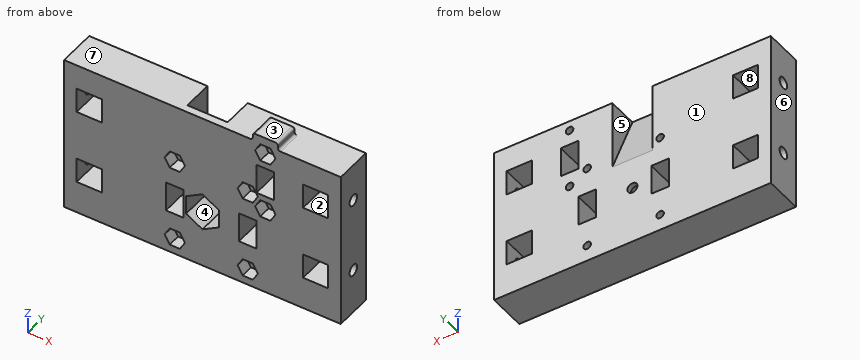
from build123d import *

# Parameters (mm, degrees)
CROQUIS1_W              = 80
CROQUIS1_H              = 60
CROQUIS1_R              = 1.5
CROQUIS1_W_2            = 7
CROQUIS1_H_2            = 25
CROQUIS1_W_3            = 10
CROQUIS1_H_3            = 20
CROQUIS1_H_4            = 10
CROQUIS1_W_4            = 5
CROQUIS1_H_5            = 6.5
SALIENTE_EXTRUIR1_DEPTH = 15
CORTAR_EXTRUIR1_DEPTH   = 5
CROQUIS3_R              = 1.5
CORTAR_EXTRUIR2_DEPTH   = 25
CROQUIS6_R              = 1.5
CORTAR_EXTRUIR3_DEPTH   = 25
CROQUIS8_W              = 15
CROQUIS8_H              = 17.838651154
CROQUIS8_R              = 2
SALIENTE_EXTRUIR2_DEPTH = 2
CORTAR_EXTRUIR4_START   = -55
CORTAR_EXTRUIR4_DEPTH   = 8
CROQUIS10_R             = 1.5
CROQUIS10_W             = 7
CROQUIS10_H             = 12
CORTAR_EXTRUIR5_DEPTH   = 16
CROQUIS12_W             = 110
CROQUIS12_H             = 15
SALIENTE_EXTRUIR3_DEPTH = 3
CORTAR_EXTRUIR6_DEPTH   = 5
SALIENTE_EXTRUIR4_DEPTH = 10
CROQUIS15_R             = 2.25
CORTAR_EXTRUIR7_DEPTH   = 10
CROQUIS16_R             = 2.25
CORTAR_EXTRUIR8_DEPTH   = 10


with BuildPart() as part:
    # Croquis1 → Saliente-Extruir1 (new body)
    with BuildSketch(Plane(origin=(0, 0, 0), x_dir=(1, 0, 0), z_dir=(0, 1, 0))):
        with Locations((0, -10)):
            Rectangle(CROQUIS1_W, CROQUIS1_H)
        with Locations(Location((18, -16.5, 0), (0, 0, 270))):
            Circle(CROQUIS1_R, mode=Mode.SUBTRACT)
        with Locations(Location((-11, -16.5, 0), (0, 0, 270))):
            Circle(CROQUIS1_R, mode=Mode.SUBTRACT)
        with Locations(Location((18, 16.5, 0), (0, 0, 270))):
            Circle(CROQUIS1_R, mode=Mode.SUBTRACT)
        with Locations(Location((-11, 16.5, 0), (0, 0, 270))):
            Circle(CROQUIS1_R, mode=Mode.SUBTRACT)
        with Locations((18, 0)):
            Rectangle(CROQUIS1_W_2, CROQUIS1_H_2, mode=Mode.SUBTRACT)
        Polygon((6.495190528, 3.75), (0, 7.5), (-6.495190528, 3.75), (-6.495190528, -3.75), (0, -7.5), (6.495190528, -3.75), align=None, mode=Mode.SUBTRACT)
        with Locations((-11, 0)):
            Rectangle(CROQUIS1_W_2, CROQUIS1_H_2, mode=Mode.SUBTRACT)
        with Locations((-45, -10)):
            Rectangle(CROQUIS1_W_3, CROQUIS1_H_3)
        with Locations((-45, -35)):
            Rectangle(CROQUIS1_W_3, CROQUIS1_H_4)
        with Locations((-52.5, -10)):
            Rectangle(CROQUIS1_W_4, CROQUIS1_H)
        with Locations((-45, 15)):
            Rectangle(CROQUIS1_W_3, CROQUIS1_H_4)
        with Locations((45, 15)):
            Rectangle(CROQUIS1_W_3, CROQUIS1_H_4)
        with Locations((52.5, -10)):
            Rectangle(CROQUIS1_W_4, CROQUIS1_H)
        with Locations((45, -10)):
            Rectangle(CROQUIS1_W_3, CROQUIS1_H_3)
        with Locations((45, -35)):
            Rectangle(CROQUIS1_W_3, CROQUIS1_H_4)
        with Locations((-11, 9.25)):
            Rectangle(CROQUIS1_W_2, CROQUIS1_H_5)
        with Locations((-11, -9.25)):
            Rectangle(CROQUIS1_W_2, CROQUIS1_H_5)
        with Locations((18, 9.25)):
            Rectangle(CROQUIS1_W_2, CROQUIS1_H_5)
        with Locations((18, -9.25)):
            Rectangle(CROQUIS1_W_2, CROQUIS1_H_5)
    extrude(amount=SALIENTE_EXTRUIR1_DEPTH)

    # Croquis2 → Cortar-Extruir1 (cut)
    with BuildSketch(Plane.XZ):
        Polygon((-6.958548116, 16.5), (-8.979274058, 20), (-13.020725942, 20), (-15.041451884, 16.5), (-13.020725942, 13), (-8.979274058, 13), align=None)
        Polygon((22.041451884, 16.5), (20.020725942, 20), (15.979274058, 20), (13.958548116, 16.5), (15.979274058, 13), (20.020725942, 13), align=None)
        Polygon((-6.958548116, -16.5), (-8.979274058, -13), (-13.020725942, -13), (-15.041451884, -16.5), (-13.020725942, -20), (-8.979274058, -20), align=None)
        Polygon((22.041451884, -16.5), (20.020725942, -13), (15.979274058, -13), (13.958548116, -16.5), (15.979274058, -20), (20.020725942, -20), align=None)
    extrude(amount=-CORTAR_EXTRUIR1_DEPTH, mode=Mode.SUBTRACT)

    # Croquis3 → Cortar-Extruir2 (cut)
    with BuildSketch(Plane(origin=(55, 0, 0), x_dir=(0, 0, -1), z_dir=(1, 0, 0))):
        with Locations((-25, 7.5)):
            Circle(CROQUIS3_R)
        with Locations((5, 7.5)):
            Circle(CROQUIS3_R)
    extrude(amount=-CORTAR_EXTRUIR2_DEPTH, mode=Mode.SUBTRACT)

    # Croquis6 → Cortar-Extruir3 (cut)
    with BuildSketch(Plane.ZY.offset(55)):
        with Locations(Location((-5, 7.5, 0), (0, 0, 180))):
            Circle(CROQUIS6_R)
        with Locations(Location((25, 7.5, 0), (0, 0, 180))):
            Circle(CROQUIS6_R)
    extrude(amount=-CORTAR_EXTRUIR3_DEPTH, mode=Mode.SUBTRACT)

    # Croquis8 → Saliente-Extruir2 (add)
    with BuildSketch(Plane(origin=(0, 15, 0), x_dir=(1, 0, 0), z_dir=(0, 1, 0))):
        Rectangle(CROQUIS8_W, CROQUIS8_H)
        with Locations(Location((0, 0, 0), (0, 0, 270))):
            Circle(CROQUIS8_R, mode=Mode.SUBTRACT)
    extrude(amount=-SALIENTE_EXTRUIR2_DEPTH)

    # Croquis9 → Cortar-Extruir4 (cut, symmetric)
    with BuildSketch(Plane(origin=(55, 0, 0), x_dir=(0, 0, -1), z_dir=(1, 0, 0)).offset(CORTAR_EXTRUIR4_START)):
        Polygon((-40, 3), (-12.5, 15), (-40, 15), align=None)
    extrude(amount=CORTAR_EXTRUIR4_DEPTH, both=True, mode=Mode.SUBTRACT)

    # Croquis10 → Cortar-Extruir5 (cut)
    with BuildSketch(Plane(origin=(0, 15, 0), x_dir=(1, 0, 0), z_dir=(0, 1, 0))):
        with Locations(Location((25, -12, 0), (0, 0, 270))):
            Circle(CROQUIS10_R)
        with Locations(Location((25, -36, 0), (0, 0, 270))):
            Circle(CROQUIS10_R)
        with Locations((25, -24)):
            Rectangle(CROQUIS10_W, CROQUIS10_H)
    extrude(amount=-CORTAR_EXTRUIR5_DEPTH, mode=Mode.SUBTRACT)

    # Croquis12 → Saliente-Extruir3 (add)
    with BuildSketch(Plane(origin=(0, 0, -20), x_dir=(-1, 0, 0), z_dir=(0, 0, -1))):
        with Locations((0, 7.5)):
            Rectangle(CROQUIS12_W, CROQUIS12_H)
    extrude(amount=SALIENTE_EXTRUIR3_DEPTH)

    # Croquis13 → Cortar-Extruir6 (cut)
    with BuildSketch(Plane.XZ):
        Polygon((29.041451884, 12), (27.020725942, 15.5), (22.979274058, 15.5), (20.958548116, 12), (22.979274058, 8.5), (27.020725942, 8.5), align=None)
        Polygon((29.041451884, 36), (27.020725942, 39.5), (22.979274058, 39.5), (20.958548116, 36), (22.979274058, 32.5), (27.020725942, 32.5), align=None)
    extrude(amount=-CORTAR_EXTRUIR6_DEPTH, mode=Mode.SUBTRACT)

    # Croquis14 → Saliente-Extruir4 (add)
    with BuildSketch(Plane.XZ):
        with BuildLine():
            Line((30, 41), (30, 42))
            ThreePointArc((30, 42), (29.707106781, 42.707106781), (29, 43))
            Line((29, 43), (21, 43))
            ThreePointArc((21, 43), (20.292893219, 42.707106781), (20, 42))
            Line((20, 42), (20, 41))
            ThreePointArc((20, 41), (19.707106781, 40.292893219), (19, 40))
            Line((19, 40), (31, 40))
            ThreePointArc((31, 40), (30.292893219, 40.292893219), (30, 41))
        make_face()
    extrude(amount=-SALIENTE_EXTRUIR4_DEPTH)

    # Croquis15 → Cortar-Extruir7 (cut)
    with BuildSketch(Plane(origin=(55, 0, 0), x_dir=(0, 0, -1), z_dir=(1, 0, 0))):
        with Locations((-25, 7.5)):
            Circle(CROQUIS15_R)
        with Locations((5, 7.5)):
            Circle(CROQUIS15_R)
    extrude(amount=-CORTAR_EXTRUIR7_DEPTH, mode=Mode.SUBTRACT)

    # Croquis16 → Cortar-Extruir8 (cut)
    with BuildSketch(Plane.ZY.offset(55)):
        with Locations(Location((-5, 7.5, 0), (0, 0, 180))):
            Circle(CROQUIS16_R)
        with Locations(Location((25, 7.5, 0), (0, 0, 180))):
            Circle(CROQUIS16_R)
    extrude(amount=-CORTAR_EXTRUIR8_DEPTH, mode=Mode.SUBTRACT)


solid = part.part
CAD build for the part. Positions are in the model's coordinates, mm. Face numbers are marked on the shaded views. A direction names the side the tool comes from. Coordinates: 2 decimals unless noted, no trailing zeros. Write each loop counter-clockwise with the first axis right and the second up, starting at its lowest first coordinate (ties: lowest second). Pieces come first, ordered by that corner, then holes. Notation, with made-up numbers: (59, -33.5) - (69, -33.5) arc R22 cw to (69, 5.5) - close; hole circle Ø11 at (5, 31). An arc over 180 degrees is marked (long way). Use a Markdown table: item, result. Add a question column.
Item 1: Drill centre lines: L1, parallel to X at y = 12.75, z = -8; L2, parallel to Z at x = 18, y = 13.25; L3, parallel to Z at x = -44, y = 5. Where is each one in solid material? Low to high. Write a range as from..to.
Item 2: Flat gauge pins, fed straight in: pin 1 (1.5 mm diameter, centred on y = 7, z = 25.5, fed in from +X); pin 2 (4 mm diameter, centred on y = 7.5, z = -5, fed in from +X); pin 3 (1.2 mm diameter, centred on x = -12, y = 3.5, fed in from +Z); pin 4 (2.5 mm diameter, centred on x = 18, z = -16.5, fed in from +Y). Where does each tip first touch, or does it go through?
Item 3: Band-saw the part on C-C, the plane x = -3.5. Give the cut face in (y, z).
Item 4: Band-saw the part on D-D, the plane x = -21. Give the cut face in (y, z).
Item 5: Band-saw the part on B-B, the plane y = 7.5. Give the number of separate pieces and of enclosed holes in the cut face, and give its area (3 significant figures).
Item 6: 3-axis set-ups, long thin cutter, end or side, ignore diameter. For the marked faces 1, 2, 3, 4 and 5: which of +Z, -Z, +X, -X, +Y, -Y reach the whole face in a straight line?
Item 7: Mould opens along X. For the marked faces 6, 7 and 8 say: pulls with the +X half, pulls with the -X half, needs draft (parallel to the pull), parting line crosses it, or undercut.
Item 8: Band-saw the part on A-A, the plane x = 25. Give the cut face in (y, z), and give its area (3 significant figures).
Numbers:
| question | item | result |
|---|---|---|
| 1 | L1 | -55..-50, -40..40, 50..55 |
| 1 | L2 | -23..-18, -15..-6, 6..15, 18..40 |
| 1 | L3 | -23..-10, 0..20, 30..40 |
| 2 | pin 1 | x = 30 |
| 2 | pin 2 | x = 40 |
| 2 | pin 3 | z = 40 |
| 2 | pin 4 | through |
| 3 | outline | (0, -23) - (15, -23) - (15, 12.5) - (3, 40) - (0, 40) - (0, 5.48) - (13, 5.48) - (13, -5.48) - (0, -5.48) - close |
| 4 | outline | (0, -23) - (15, -23) - (15, 40) - (0, 40) - close |
| 5 | separate pieces | 1 |
| 5 | enclosed holes | 10 |
| 5 | area | 5,740 mm2 |
| 6 | face 1 | +Z, -Z, +X, -X, +Y |
| 6 | face 2 | +Y, -Y |
| 6 | face 3 | +Z, +X, -X, +Y, -Y |
| 6 | face 4 | -Y |
| 6 | face 5 | +Z, +Y |
| 7 | face 6 | pulls with the -X half |
| 7 | face 7 | needs draft |
| 7 | face 8 | undercut |
| 8 | outline | (0, -23) - (15, -23) - (15, 10.5) - (5, 10.5) - (5, 8.5) - (0, 8.5) - close; (0, 15.5) - (5, 15.5) - (5, 13.5) - (15, 13.5) - (15, 18) - (0, 18) - close; (0, 30) - (15, 30) - (15, 34.5) - (5, 34.5) - (5, 32.5) - (0, 32.5) - close; (0, 39.5) - (5, 39.5) - (5, 37.5) - (15, 37.5) - (15, 40) - (10, 40) - (10, 43) - (0, 43) - close |
| 8 | area | 665 mm2 |
